Read the model definition and answer for the solid it produces. Units are mm, in the model's axes. Face numbers are marked on the shaded views. A direction names the side the tool comes from. Give positions to 0.01 mm unless a question says otherwise; leave off trailing zeros. Write each loop counter-clockwise with the first axis right and the second up, starting at its lowest first coordinate (ties: lowest second). Pieces come first, ordered by that corner, then holes.
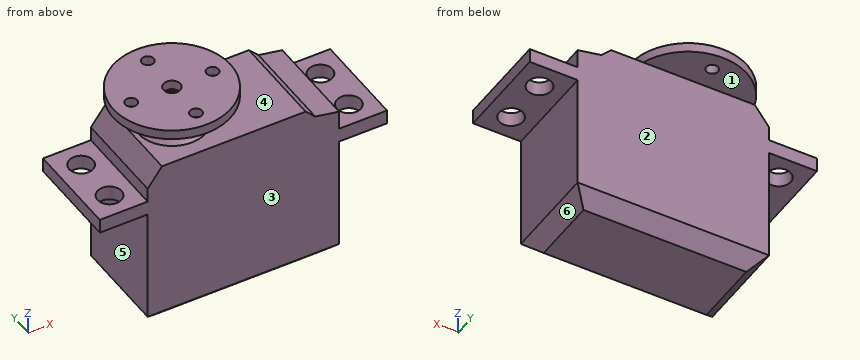
```python
from build123d import *

# Parameters (mm, degrees)
SKETCH_1_W             = 40
SKETCH_1_H             = 20
EXTRUDE_1_DEPTH        = 37
CUT_EXTRUDE_1_DEPTH    = 47.572524089
CUT_EXTRUDE_2_DEPTH    = 47.572524089
CHAMFER_1_SIZE         = 3
SKETCH_4_R             = 7
EXTRUDE_2_DEPTH        = 2
CHAMFER_2_SIZE         = 2
SKETCH_5_R             = 3
EXTRUDE_3_DEPTH        = 4
SKETCH_6_W             = 10
SKETCH_6_H             = 20
EXTRUDE_4_DEPTH        = 3
SKETCH_7_R             = 2.5
CUT_EXTRUDE_3_DEPTH    = 3
HOLE_WIZARD_M3_1_D     = 2.5
HOLE_WIZARD_M3_1_DEPTH = 8.5
HOLE_WIZARD_M3_1_TIP   = 0.751075774
SKETCH_10_R            = 12.25
SKETCH_10_R_2          = 1.25
SKETCH_10_R_3          = 1.75
EXTRUDE_5_DEPTH        = 2


with BuildPart() as part:
    # 草图1 → 凸台-拉伸1 (new body)
    with BuildSketch(Plane.XY):
        Rectangle(SKETCH_1_W, SKETCH_1_H)
    extrude(amount=EXTRUDE_1_DEPTH)

    # 草图2 → 切除-拉伸1 (cut, through all)
    with BuildSketch(Plane.XZ.offset(10)):
        Polygon((20, 34), (15, 35), (13, 37), (20, 37), align=None)
    extrude(amount=-CUT_EXTRUDE_1_DEPTH, mode=Mode.SUBTRACT)

    # 草图3 → 切除-拉伸2 (cut, through all)
    with BuildSketch(Plane.XZ.offset(10)):
        Polygon((-20, 37), (-17, 37), (-20, 33), align=None)
    extrude(amount=-CUT_EXTRUDE_2_DEPTH, mode=Mode.SUBTRACT)

    # 倒角1
    chamfer_1_edges = [part.edges().sort_by_distance(p)[0] for p in [
        (0, -10, 0),
        (-20, 0, 0),
        (0, 10, 0),
        (20, 0, 0),
    ]]
    chamfer(chamfer_1_edges, length=CHAMFER_1_SIZE)

    # 草图4 → 凸台-拉伸2 (add)
    with BuildSketch(Plane.XY.offset(37)):
        with Locations(Location((-9, 0, 0), (0, 0, 180))):
            Circle(SKETCH_4_R)
    extrude(amount=EXTRUDE_2_DEPTH)

    # 倒角2
    chamfer_2_edges = [part.edges().sort_by_distance(p)[0] for p in [
        (-2, 0, 39),
    ]]
    chamfer(chamfer_2_edges, length=CHAMFER_2_SIZE - 0.0001)  # a hair under: the kernel refuses the full size

    # 草图5 → 凸台-拉伸3 (add)
    with BuildSketch(Plane.XY.offset(39)):
        with Locations((-9, 0)):
            Circle(SKETCH_5_R)
    extrude(amount=EXTRUDE_3_DEPTH)

    # 草图6 → 凸台-拉伸4 (add)
    with BuildSketch(Plane(origin=(0, 0, 30), x_dir=(-1, 0, 0), z_dir=(0, 0, -1))):
        with Locations((25, 0)):
            Rectangle(SKETCH_6_W, SKETCH_6_H)
        with Locations((-25, 0)):
            Rectangle(SKETCH_6_W, SKETCH_6_H)
    extrude(amount=EXTRUDE_4_DEPTH)

    # 草图7 → 切除-拉伸3 (cut)
    with BuildSketch(Plane.XY.offset(30)):
        with Locations((-25, 5)):
            Circle(SKETCH_7_R)
        with Locations((-25, -5)):
            Circle(SKETCH_7_R)
    cut_extrude_3 = extrude(amount=-CUT_EXTRUDE_3_DEPTH, mode=Mode.SUBTRACT)

    # 镜向1: 切除-拉伸3 across plane
    add(cut_extrude_3.mirror(Plane(origin=(0, 0, 0), x_dir=(0, 0, 1), z_dir=(1, 0, 0))), mode=Mode.SUBTRACT)

    # M3 螺纹孔1
    with Locations(Plane.XY.offset(43)):
        with Locations((-9, 0)):
            Hole(HOLE_WIZARD_M3_1_D / 2, depth=HOLE_WIZARD_M3_1_DEPTH)
            with Locations((0, 0, -(HOLE_WIZARD_M3_1_DEPTH + HOLE_WIZARD_M3_1_TIP / 2))):  # 118° drill point
                Cone(0, HOLE_WIZARD_M3_1_D / 2, HOLE_WIZARD_M3_1_TIP, mode=Mode.SUBTRACT)

    # 草图10 → 凸台-拉伸5 (add)
    with BuildSketch(Plane.XY.offset(43)):
        with Locations((-9, 0)):
            Circle(SKETCH_10_R)
        with Locations((-9, 8.5)):
            Circle(SKETCH_10_R_2, mode=Mode.SUBTRACT)
        with Locations((-0.5, 0)):
            Circle(SKETCH_10_R_2, mode=Mode.SUBTRACT)
        with Locations((-9, -8.5)):
            Circle(SKETCH_10_R_2, mode=Mode.SUBTRACT)
        with Locations((-17.5, 0)):
            Circle(SKETCH_10_R_2, mode=Mode.SUBTRACT)
        with Locations((-9, 0)):
            Circle(SKETCH_10_R_3, mode=Mode.SUBTRACT)
    extrude(amount=EXTRUDE_5_DEPTH)


solid = part.part
```
Item 1: Each of these flat-tipped pins is pushed along its axis until it touches: pin 1 Ø5 at (x, y) = (-26.5, -1) entering from -Z; pin 2 Ø12 at (y, z) = (2, 17.5) entering from +X; pin 3 Ø5 at (y, z) = (-3, 23) entering from -X; pin 4 Ø4.5 at (x, y) = (-25, 5) entering from +Z (3 decimals). Where does it stop, or does it pass through?
Result set:
pin 1: stops at z = 27
pin 2: stops at x = 20
pin 3: stops at x = -20
pin 4: passes through
Item 2: Which of the six approach directions +Z, -Z, +X, -X, +Y, -Y give full straight-line access (tool end or side, diameter ignored) to the marked faces 1, 2 and 3?
Result set:
face 1: none
face 2: -Z, +X, -X, +Y
face 3: -Z, +X, -X, -Y
Item 3: Section C-C (z = 41.5) is taken. Write down the section's boundary in (x, y), and give its area (3 significant figures).
Result set:
outline: circle Ø6 at (-9, 0); hole circle Ø2.5 at (-9, 0)
area: 23.4 mm2
Item 4: Section A-A (x = 25) is taken. Write down the section's boundary in (y, z), and give its area (3 significant figures).
Result set:
outline: (-10, 27) - (-7.5, 27) - (-7.5, 30) - (-10, 30) - close; (-2.5, 27) - (2.5, 27) - (2.5, 30) - (-2.5, 30) - close; (7.5, 27) - (10, 27) - (10, 30) - (7.5, 30) - close
area: 30.0 mm2
Item 5: Find the intervals of material crossed by line 1 along Y through (x, z) = (25, 28); line 2 along Z through (x, y) = (-1.5, -1); line 3 along X through (y, z) = (8.25, 12.5), in increasing order.
Result set:
line 1: y = -10 to -7.5, -2.5 to 2.5, 7.5 to 10
line 2: z = 0 to 37, 43 to 45
line 3: x = -20 to 20
Item 6: Determine the mould class of the marked faces 4, 5 and 6 for opening direction Z: pulls with the +Z half, pulls with the -Z half, needs draft (parallel to the pull), parting line crosses it, or undercut.
Result set:
face 4: undercut
face 5: needs draft
face 6: pulls with the -Z half
Item 7: Section B-B (y = -8.5) is taken. Write down the section's boundary in (x, z).
Result set:
outline: (-30, 27) - (-20, 27) - (-20, 3) - (-18.5, 1.5) - (18.5, 1.5) - (20, 3) - (20, 27) - (30, 27) - (30, 30) - (20, 30) - (20, 34) - (15, 35) - (13, 37) - (-17, 37) - (-20, 33) - (-20, 30) - (-30, 30) - close; (-17.82, 43) - (-10.25, 43) - (-10.25, 45) - (-17.82, 45) - close; (-7.75, 43) - (-0.18, 43) - (-0.18, 45) - (-7.75, 45) - close
